CAD build for the part. Positions are in the model's coordinates, mm. A direction names the side the tool comes from. Round coordinates to 2 decimals unless told otherwise and drop trailing zeros. Loops run counter-clockwise (first coordinate to the right, second up) from the corner with the lowest first, then second, coordinate; pieces in that order, holes last.
Autodesk Inventor part; units mm, degrees
ref_plane "Start Plane" through (0, 0, 0) normal (0, 0, 1) x (1, 0, 0)
ref_plane "End Plane" through (0, 0, 63.5) normal (0, 0, 1) x (1, 0, 0)
ref_plane "YZ Plane" through (0, 0, 0) normal (1, 0, 0) x (0, 1, 0)
ref_plane "Start Plane" through (0, 0, 0) normal (0, 0, 1) x (1, 0, 0)
ref_plane "End Plane" through (0, 0, 63.5) normal (0, 0, 1) x (1, 0, 0)
sketch "Sketch" plane through (0, 0, 0) normal (0, 0, 1) x (1, 0, 0)
  arc A0 (-11.6332, 12.7) -> (-12.7, 11.6332) centre (-11.6332, 11.6332) ccw
  arc A1 (-5.3594, 10.5664) -> (-5.3594, 12.7) centre (-5.3594, 11.6332) ccw
  arc A2 (-12.7, 5.3594) -> (-10.5664, 5.3594) centre (-11.6332, 5.3594) ccw
  line L0 (-10.5664, 7.493) -> (-10.5664, 5.3594)
  line L1 (-7.493, 10.5664) -> (-5.3594, 10.5664)
  arc A3 (-9.6992, 7.8522) -> (-10.5664, 7.493) centre (-10.0584, 7.493) ccw
  arc A4 (-7.493, 10.5664) -> (-7.8522, 9.6992) centre (-7.493, 10.0584) ccw
  line L2 (-11.6332, 11.6332) -> (0, 0) construction
  line L3 (-5.8003, 3.9533) -> (-9.6992, 7.8522)
  line L4 (-7.8522, 9.6992) -> (-3.9533, 5.8003)
  arc A5 (-3.9533, 5.8003) -> (-2.6924, 5.278) centre (-2.6924, 7.0612) ccw
  arc A6 (-5.278, 2.6924) -> (-5.8003, 3.9533) centre (-7.0612, 2.6924) ccw
  arc A7 (0, 2.54) -> (-2.54, 0) centre (0, 0) ccw construction
  line L5 (0, 0) -> (-12.7, 0) construction
  line L6 (0, 12.7) -> (0, 0) construction
  arc A8 (-11.6332, 12.7) -> (-10.6172, 12.7) centre (-11.1252, 12.7) ccw
  arc A9 (-7.5692, 12.7) -> (-6.5532, 12.7) centre (-7.0612, 12.7) ccw
  arc A10 (-12.7, 10.6172) -> (-12.7, 11.6332) centre (-12.7, 11.1252) ccw
  arc A11 (-12.7, 6.5532) -> (-12.7, 7.5692) centre (-12.7, 7.0612) ccw
  line L7 (-12.7, 10.6172) -> (-12.7, 7.5692)
  line L8 (-12.7, 6.5532) -> (-12.7, 5.3594)
  line L9 (-10.6172, 12.7) -> (-7.5692, 12.7)
  line L10 (-6.5532, 12.7) -> (-5.3594, 12.7)
  circle A12 centre (0, 0) radius 2.54
  arc A13 (-12.7, -11.6332) -> (-11.6332, -12.7) centre (-11.6332, -11.6332) ccw
  line L11 (-12.7, -10.6172) -> (-12.7, -7.5692)
  arc A14 (-10.5664, -7.493) -> (-9.6992, -7.8522) centre (-10.0584, -7.493) ccw
  line L12 (-9.6992, -7.8522) -> (-5.8003, -3.9533)
  line L13 (-11.6332, -11.6332) -> (0, 0) construction
  line L14 (-3.9533, -5.8003) -> (-7.8522, -9.6992)
  arc A15 (-7.8522, -9.6992) -> (-7.493, -10.5664) centre (-7.493, -10.0584) ccw
  line L15 (-10.6172, -12.7) -> (-7.5692, -12.7)
  line L16 (-7.493, -10.5664) -> (-5.3594, -10.5664)
  arc A16 (-6.5532, -12.7) -> (-7.5692, -12.7) centre (-7.0612, -12.7) ccw
  line L17 (-6.5532, -12.7) -> (-5.3594, -12.7)
  arc A17 (-5.3594, -12.7) -> (-5.3594, -10.5664) centre (-5.3594, -11.6332) ccw
  arc A18 (-10.6172, -12.7) -> (-11.6332, -12.7) centre (-11.1252, -12.7) ccw
  arc A19 (-12.7, -11.6332) -> (-12.7, -10.6172) centre (-12.7, -11.1252) ccw
  arc A20 (-2.6924, -5.278) -> (-3.9533, -5.8003) centre (-2.6924, -7.0612) ccw
  arc A21 (-5.8003, -3.9533) -> (-5.278, -2.6924) centre (-7.0612, -2.6924) ccw
  line L18 (-10.5664, -7.493) -> (-10.5664, -5.3594)
  line L19 (-12.7, -6.5532) -> (-12.7, -5.3594)
  arc A22 (-10.5664, -5.3594) -> (-12.7, -5.3594) centre (-11.6332, -5.3594) ccw
  arc A23 (-12.7, -7.5692) -> (-12.7, -6.5532) centre (-12.7, -7.0612) ccw
  arc A24 (11.6332, -12.7) -> (12.7, -11.6332) centre (11.6332, -11.6332) ccw
  line L20 (10.6172, -12.7) -> (7.5692, -12.7)
  arc A25 (7.493, -10.5664) -> (7.8522, -9.6992) centre (7.493, -10.0584) ccw
  line L21 (7.8522, -9.6992) -> (3.9533, -5.8003)
  line L22 (11.6332, -11.6332) -> (0, 0) construction
  line L23 (5.8003, -3.9533) -> (9.6992, -7.8522)
  arc A26 (9.6992, -7.8522) -> (10.5664, -7.493) centre (10.0584, -7.493) ccw
  line L24 (12.7, -10.6172) -> (12.7, -7.5692)
  line L25 (10.5664, -7.493) -> (10.5664, -5.3594)
  arc A27 (12.7, -6.5532) -> (12.7, -7.5692) centre (12.7, -7.0612) ccw
  line L26 (12.7, -6.5532) -> (12.7, -5.3594)
  arc A28 (12.7, -5.3594) -> (10.5664, -5.3594) centre (11.6332, -5.3594) ccw
  arc A29 (12.7, -10.6172) -> (12.7, -11.6332) centre (12.7, -11.1252) ccw
  arc A30 (11.6332, -12.7) -> (10.6172, -12.7) centre (11.1252, -12.7) ccw
  arc A31 (5.278, -2.6924) -> (5.8003, -3.9533) centre (7.0612, -2.6924) ccw
  arc A32 (3.9533, -5.8003) -> (2.6924, -5.278) centre (2.6924, -7.0612) ccw
  line L27 (7.493, -10.5664) -> (5.3594, -10.5664)
  line L28 (6.5532, -12.7) -> (5.3594, -12.7)
  arc A33 (5.3594, -10.5664) -> (5.3594, -12.7) centre (5.3594, -11.6332) ccw
  arc A34 (7.5692, -12.7) -> (6.5532, -12.7) centre (7.0612, -12.7) ccw
  arc A35 (12.7, 11.6332) -> (11.6332, 12.7) centre (11.6332, 11.6332) ccw
  line L29 (12.7, 10.6172) -> (12.7, 7.5692)
  arc A36 (10.5664, 7.493) -> (9.6992, 7.8522) centre (10.0584, 7.493) ccw
  line L30 (9.6992, 7.8522) -> (5.8003, 3.9533)
  line L31 (11.6332, 11.6332) -> (0, 0) construction
  line L32 (3.9533, 5.8003) -> (7.8522, 9.6992)
  arc A37 (7.8522, 9.6992) -> (7.493, 10.5664) centre (7.493, 10.0584) ccw
  line L33 (10.6172, 12.7) -> (7.5692, 12.7)
  line L34 (7.493, 10.5664) -> (5.3594, 10.5664)
  arc A38 (6.5532, 12.7) -> (7.5692, 12.7) centre (7.0612, 12.7) ccw
  line L35 (6.5532, 12.7) -> (5.3594, 12.7)
  arc A39 (5.3594, 12.7) -> (5.3594, 10.5664) centre (5.3594, 11.6332) ccw
  arc A40 (10.6172, 12.7) -> (11.6332, 12.7) centre (11.1252, 12.7) ccw
  arc A41 (12.7, 11.6332) -> (12.7, 10.6172) centre (12.7, 11.1252) ccw
  arc A42 (2.6924, 5.278) -> (3.9533, 5.8003) centre (2.6924, 7.0612) ccw
  arc A43 (5.8003, 3.9533) -> (5.278, 2.6924) centre (7.0612, 2.6924) ccw
  line L36 (10.5664, 7.493) -> (10.5664, 5.3594)
  line L37 (12.7, 6.5532) -> (12.7, 5.3594)
  arc A44 (10.5664, 5.3594) -> (12.7, 5.3594) centre (11.6332, 5.3594) ccw
  arc A45 (12.7, 7.5692) -> (12.7, 6.5532) centre (12.7, 7.0612) ccw
  line L38 (-2.6924, 5.278) -> (2.6924, 5.278)
  line L39 (-5.278, 2.6924) -> (-5.278, -2.6924)
  line L40 (-2.6924, -5.278) -> (2.6924, -5.278)
  line L41 (5.278, -2.6924) -> (5.278, 2.6924)
  point P0 (0, 0)
  point P1 (0, 0)
  dimension "d2" = 2.1336
  dimension "d3" = 6.2738
  dimension "d4" = 6.2738
  dimension "d5" = 1.0668
  dimension "d6" = 2.1336
  dimension "d7" = 2.1336
  dimension "d8" = 1.016
  dimension "d9" = 1.016
  dimension "d10" = 135
  dimension "d11" = 2.667
  dimension "d12" = 4.572
  dimension "d13" = 4.572
  dimension "d14" = 2.667
  dimension "d15" = 5.08
  dimension "d16" = 45
  dimension "d19" = 45
  dimension "d20" = 0.508
  dimension "d21" = 4.572
  dimension "d22" = 1.016
  dimension "d23" = 4.572
  dimension "d24" = 1.016
  dimension "d25" = 0.508
  dimension "d26" = 0.508
  dimension "d27" = 0.508
  dimension "d28" = 12.7
  dimension "d37" = 360
  dimension "d47" = 10.5664
  dimension "d48" = 12.7
extrude "Body" add sketch "Sketch" along normal up to surface (63.5 mm away) from surface at 0
sketch "Sketch4" plane through (0, 0, 0) normal (0, 0, 1) x (1, 0, 0)
  line L0 (0, 0) -> (10, 0)
ref_plane "Work Plane4" through (0, 0, 0) normal (0, -1, 0) x (1, 0, 0)
sketch "Sketch5" plane through (0, 0, 0) normal (0, -1, 0) x (1, 0, 0)
  line L0 (-2, 0) -> (12, 0)
  line L1 (-2, 63.5) -> (12, 63.5)
  dimension "d60" = 63.5
equation "\"d3\" = d4"
equation "\"d6\" = d7"
equation "\"d11\" = d14"
equation "\"d12\" = d13"
equation "\"d23\" = d21"
equation "\"d24\" = d30"
equation "\"d26\" = 0.5 * d24"
equation "\"d27\" = 0.5 * d22"
equation "\"Width\" = 2 * d28"
equation "\"Height\" = 2 * d48"
equation "\"G_OFFSET_START\" = 0"
equation "\"G_OFFSET_END\" = 0"
equation "\"d56\" = Length + G_OFFSET_END"
equation "\"G_L\" = 63.5"
properties part number "1010_80_20" material "Aluminum-6061"
Item 1: Wall check: L1, parallel to Y at x = 11.75, z = 14; L2, parallel to Y at x = 0, z = 48; L3, parallel to Y at x = -7.25, z = 48. Give the ranges that are in metal, low to high.
Verdict:
L1: y = -12.69 to -4.3, 4.3 to 12.69
L2: y = -5.28 to -2.54, 2.54 to 5.28
L3: y = -12.23 to -10.57, -9.1 to -5.4, 5.4 to 9.1, 10.57 to 12.23
Item 2: 3-axis set-ups, long thin cutter, end or side, ignore diameter. For faces 4 (the flat face through (0, 5.278, 31)), 5 (the flat face through (10.566, 6, 31)), 6 (the cylindrical face through (-5.418, 3.384, 31.306)): which of +Z, -Z, +X, -X, +Y, -Y reach the whole face in a straight line?
Verdict:
face 4: +Z, -Z, +Y
face 5: +Z, -Z
face 6: +Z, -Z, -X
Item 3: Flat gauge pins, fed straight in: P1, Ø2.5, axis at x = 0.5, z = 24, coming from the +Y side; P2, Ø2.5, axis at x = 0.5, z = 27.5, coming from the -Y side; P3, Ø4.5, axis at y = -0.5, z = 36.5, coming from the +X side; P4, Ø2, axis at x = 10, y = -3.5, coming from the -Z side. Where does each tip first touch, or does it go through?
Verdict:
P1: stops at y = 5.28
P2: stops at y = -5.28
P3: stops at x = 5.28
P4: passes through
Item 4: Cut at A-A (y = 0). List the corners of the cut face in (x, z).
Verdict:
outline: (-5.28, 0) - (-2.54, 0) - (-2.54, 63.5) - (-5.28, 63.5) - close; (2.54, 0) - (5.28, 0) - (5.28, 63.5) - (2.54, 63.5) - close
Item 5: Mould opens along Y. For faces 1 (the flat face through (-12.7, 9, 31)), 2 (the flat face through (-6, 10.566, 31)), 3 (the cylindrical face through (-3.37, 5.41, 31.31)) say: released by +Y, released by -Y, zero draft, split by the parting line, or undercut.
Verdict:
face 1: zero draft
face 2: undercut
face 3: released by +Y
